The model under review builds one solid part; all positions refer to its coordinate system, in mm. Face numbers are marked on the shaded views. A direction names the side the tool comes from. Coordinates: 2 decimals unless noted, no trailing zeros. Order: outer loops, then holes, each group sorted by start corner. A loop starts at its lowest first (then second) coordinate and runs counter-clockwise, first axis right, second up.
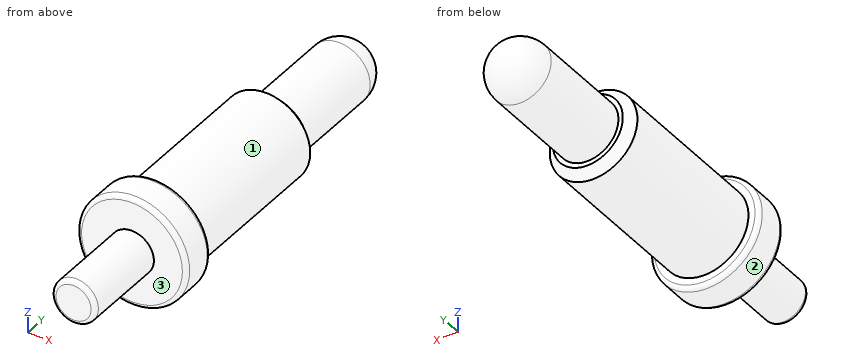
```python
from build123d import *

# Parameters (mm, degrees)
SKETCH_1_R      = 0.5
EXTRUDE_1_DEPTH = 2
SKETCH_2_R      = 1.25
EXTRUDE_2_DEPTH = 0.8
SKETCH_3_R      = 1
EXTRUDE_3_DEPTH = 4
SKETCH_4_R      = 0.7
EXTRUDE_4_DEPTH = 3
FILLET_1_R      = 0.7
CHAMFER_1_SIZE  = 0.2
FILLET_2_R      = 0.1


with BuildPart() as part:
    # 草图1 → 凸台-拉伸1 (new body)
    with BuildSketch(Plane(origin=(0, 0, 0), x_dir=(1, 0, 0), z_dir=(0, 1, 0))):
        Circle(SKETCH_1_R)
    extrude(amount=-EXTRUDE_1_DEPTH)

    # 草图2 → 凸台-拉伸2 (add)
    with BuildSketch(Plane(origin=(0, 0, 0), x_dir=(1, 0, 0), z_dir=(0, 1, 0))):
        Circle(SKETCH_2_R)
    extrude(amount=EXTRUDE_2_DEPTH)

    # 草图3 → 凸台-拉伸3 (add)
    with BuildSketch(Plane(origin=(0, 0.8, 0), x_dir=(1, 0, 0), z_dir=(0, 1, 0))):
        Circle(SKETCH_3_R)
    extrude(amount=EXTRUDE_3_DEPTH)

    # 草图4 → 凸台-拉伸4 (add)
    with BuildSketch(Plane(origin=(0, 4.8, 0), x_dir=(1, 0, 0), z_dir=(0, 1, 0))):
        Circle(SKETCH_4_R)
    extrude(amount=EXTRUDE_4_DEPTH)

    # 圆角1
    fillet_1_edges = [part.edges().sort_by_distance(p)[0] for p in [
        (-0.7, 7.8, 0),
    ]]
    fillet(fillet_1_edges, radius=FILLET_1_R)

    # 倒角1
    chamfer_1_edges = [part.edges().sort_by_distance(p)[0] for p in [
        (-1, 4.8, 0),
    ]]
    chamfer(chamfer_1_edges, length=CHAMFER_1_SIZE)

    # 圆角2
    fillet_2_edges = [part.edges().sort_by_distance(p)[0] for p in [
        (-0.5, -2, 0),
        (-1.25, 0, 0),
        (-1.25, 0.8, 0),
    ]]
    fillet(fillet_2_edges, radius=FILLET_2_R)


solid = part.part
```
(1) Wall thickness on probe 1 along X at (y, z) = (3.25, 0.6); probe 2 along Y at (x, z) = (-0.5, 0.6); probe 3 along Z at (x, y) = (0, 2.25): over which ranges is each line inside the solid? List them lowest first.
A:
probe 1: x = -0.8 to 0.8
probe 2: y = 0 to 4.8
probe 3: z = -1 to 1
(2) We need section A-A, the plane z = 0. Write out the cut boundary in (x, y), and give its area (3 significant figures).
A:
outline: (-1.25, 0.1) arc R0.1 ccw to (-1.15, 0) - (-0.5, 0) - (-0.5, -1.9) arc R0.1 ccw to (-0.4, -2) - (0.4, -2) arc R0.1 ccw to (0.5, -1.9) - (0.5, 0) - (1.15, 0) arc R0.1 ccw to (1.25, 0.1) - (1.25, 0.7) arc R0.1 ccw to (1.15, 0.8) - (1, 0.8) - (1, 4.6) - (0.8, 4.8) - (0.7, 4.8) - (0.7, 7.1) arc R0.7 ccw to (-0.7, 7.1) - (-0.7, 4.8) - (-0.8, 4.8) - (-1, 4.6) - (-1, 0.8) - (-1.15, 0.8) arc R0.1 ccw to (-1.25, 0.7) - close
area: 15.9 mm2
(3) We need section B-B, the plane x = 0. Write out the cut boundary in (y, z).
A:
outline: (-2, -0.4) arc R0.1 ccw to (-1.9, -0.5) - (0, -0.5) - (0, -1.15) arc R0.1 ccw to (0.1, -1.25) - (0.7, -1.25) arc R0.1 ccw to (0.8, -1.15) - (0.8, -1) - (4.6, -1) - (4.8, -0.8) - (4.8, -0.7) - (7.1, -0.7) arc R0.7 ccw to (7.1, 0.7) - (4.8, 0.7) - (4.8, 0.8) - (4.6, 1) - (0.8, 1) - (0.8, 1.15) arc R0.1 ccw to (0.7, 1.25) - (0.1, 1.25) arc R0.1 ccw to (0, 1.15) - (0, 0.5) - (-1.9, 0.5) arc R0.1 ccw to (-2, 0.4) - close
(4) We need section D-D, the plane y = 2.5. Write out the cut boundary in (x, z).
A:
outline: circle Ø2 at (0, 0)
(5) We need section C-C, the plane y = -1. Write out the cut boundary in (x, z).
A:
outline: circle Ø1 at (0, 0)
(6) For pin 1 Ø1 at (x, y) = (0, 5) entering from +Z, flat-tipped, find the tip position at first contact; note if it passes through.
A:
pin 1: stops at z = 1
(7) Machinability: for the marked faces 1, 2 and 3, which of the approach directions +Z, -Z, +X, -X, +Y, -Y give a long, thin tool a straight path to every point of the face, cutting with its end or side? Answer none if there is none.
A:
face 1: +Y
face 2: +Y, -Y
face 3: -Y
